Verification items for this drawing (mm, ordinates from the low corner). A direction names the side the tool comes from. Give positions to 0.01 mm unless a question says otherwise; leave off trailing zeros. Write each loop counter-clockwise with the first axis right and the second up, starting at its lowest first coordinate (ties: lowest second). Pieces come first, ordered by that corner, then holes. Notation, with made-up numbers: (50, 14) -> (64, 14) arc R30 ccw to (64, 45) -> close; hole circle Ø7 at (73, 28). An arc over 180 degrees is marked (long way). Use one line per item in the form item = value. Start each with the question number.
(1) Section check B-B, the plane x = 19. Record the cut outline in (y, z), plus the area to 3 significant figures.
(2) Section check D-D, the plane z = 40. Record the cut outline in (x, y).
(3) Scan lines: L1, parallel to Z at x = 47.5, y = 10.5 (1 decimal); L2, parallel to Z at x = 59.3, y = 11.4; L3, parallel to Y at x = 21.5, z = 110.5. Record each from-to range of solid material in increasing order.
(4) Set-up check for the marked faces 1 and 2: record each of +Z, -Z, +X, -X, +Y, -Y from which the full face is reachable in a straight line by a thin tool's end or side.
(5) Section check C-C, the plane y = 13.5. State how many separate pieces and enclosed holes the cut face has, plus the area to 3 significant figures.
(6) Section check A-A, the plane z = 60. Record the cut outline in (x, y).
(7) Depth check by flat-ended pin: pin 1 Ø1.5 at (x, y) = (56, 7.5) entering from +Z; pin 2 Ø1.5 at (x, y) = (53.5, 7) entering from -Z; pin 3 Ø2.5 at (y, z) = (7.5, 74) entering from +X. Enter the tip coordinate at first touch or a pass-through.
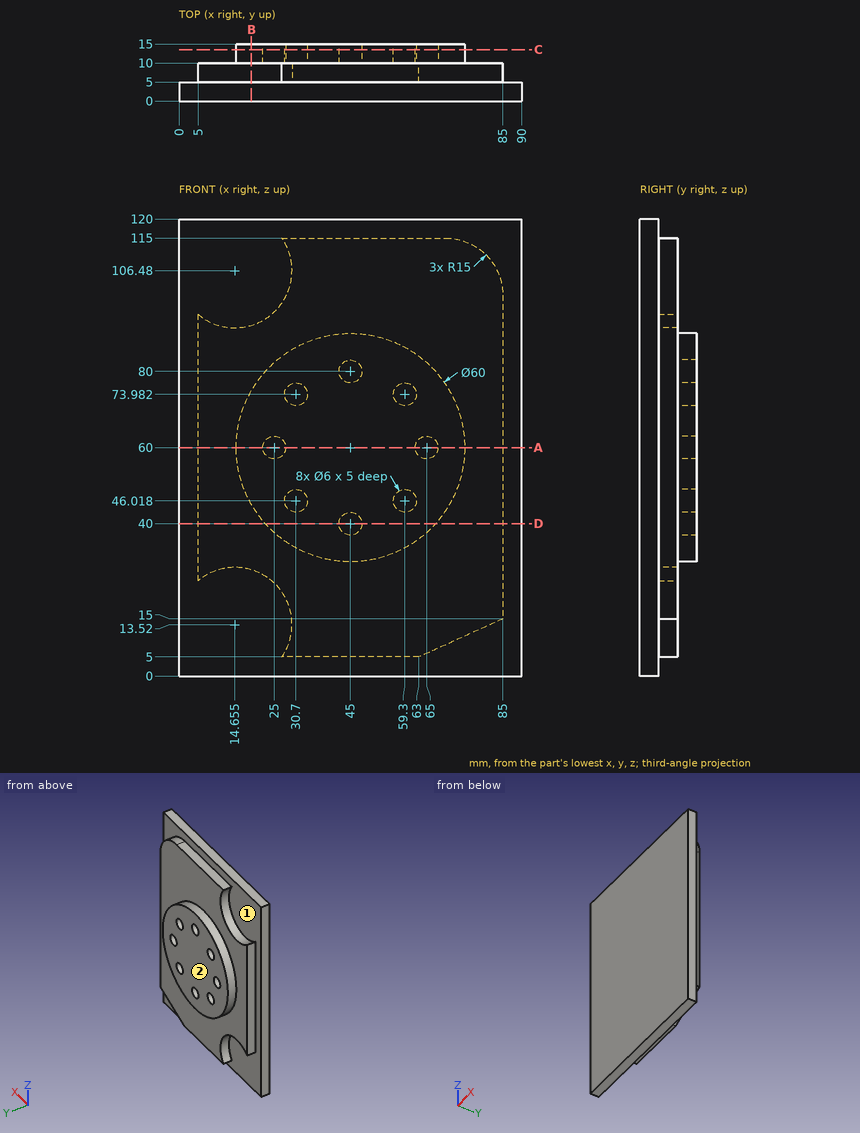
Completed:
q1.outline = (0, 0) -> (5, 0) -> (5, 27.88) -> (10, 27.88) -> (10, 45.03) -> (15, 45.03) -> (15, 74.97) -> (10, 74.97) -> (10, 92.12) -> (5, 92.12) -> (5, 120) -> (0, 120) -> close
q1.area = 1,070 mm²
q2.outline = (0, 0) -> (90, 0) -> (90, 5) -> (85, 5) -> (85, 10) -> (67.36, 10) -> (67.36, 15) -> (48, 15) -> (48, 10) -> (42, 10) -> (42, 15) -> (22.64, 15) -> (22.64, 10) -> (5, 10) -> (5, 5) -> (0, 5) -> close
q3.L1 = 30.1 to 38.3, 41.7 to 78.3, 81.7 to 89.9
q3.L2 = 33.63 to 43.02, 49.02 to 70.98, 76.98 to 86.37
q3.L3 = 0 to 5
q4.face_1 = +Y
q4.face_2 = +Z, -Z, +X, -X, +Y
q5.separate_pieces = 1
q5.enclosed_holes = 8
q5.area = 2,600 mm²
q6.outline = (0, 0) -> (90, 0) -> (90, 5) -> (85, 5) -> (85, 10) -> (75, 10) -> (75, 15) -> (68, 15) -> (68, 10) -> (62, 10) -> (62, 15) -> (28, 15) -> (28, 10) -> (22, 10) -> (22, 15) -> (15, 15) -> (15, 10) -> (5, 10) -> (5, 5) -> (0, 5) -> close
q7.pin_1 = 115
q7.pin_2 = 5
q7.pin_3 = 85
